Source: CAD feature listing. Evaluate the final solid. Frame: model axes, mm. Face numbers are marked on the shaded views. Coordinates: 2 decimals unless noted, no trailing zeros. Loops run counter-clockwise (first coordinate to the right, second up) from the corner with the lowest first, then second, coordinate; pieces in that order, holes last. Notation, with made-up numbers: M 41.25,74.5 L 60.25,74.5 A18 cw 60.25,81.5 Z; hole C 42.5,-36.5 d3. An arc over 180 degrees is marked long. One line per question, with ' | ' between items. Start each with the question number.
1. Mould query, pull axis Y, two halves, no side actions, for the marked faces 1, 2 and 3. Classes: pulls with the +Y half, pulls with the -Y half, needs draft (parallel to the pull), parting line crosses it, or undercut.
2. Section query B-B, the plane y = 136. Output: boundary loops of the cut face in (x, z).
3. Ray query, probe 1 along Z at (x, y) = (2, 156); probe 2 along X at (y, z) = (58.5, 8.5); probe 3 along Z at (x, y) = (-29.5, 100). Return the intervals inside material, ascending.
4. Pin query (flat end, axial travel): P1, Ø1.5, axis at x = 0.5, z = -1, coming from the -Y side; P2, Ø15, axis at x = 5.5, z = -7.5, coming from the -Y side; P3, Ø4, axis at x = 4.5, y = 189, coming from the +Z side. Return the tip coordinate at first contact, or that it passes through.
5. Section query A-A, the plane y = 266. Output: boundary loops of the cut face in (x, z), and give its area (3 significant figures).
Autodesk Inventor part; units mm, degrees
ref_plane "YZ Plane" through (0, 0, 0) normal (1, 0, 0) x (0, 1, 0)
ref_plane "XZ Plane" through (0, 0, 0) normal (0, 1, 0) x (-1, 0, 0)
ref_plane "XY Plane" through (0, 0, 0) normal (0, 0, 1) x (1, 0, 0)
sketch "Boceto1" plane through (0, 0, 0) normal (0, 0, 1) x (1, 0, 0)
  point P0 (0, 0)
sketch "Boceto2" plane through (0, 0, 0) normal (0, 1, 0) x (-1, 0, 0)
  point P0 (0, 0)
sketch "Boceto3" plane through (0, 0, 0) normal (0, 1, 0) x (-1, 0, 0)
  circle A0 centre (0, 0) radius 37.5
  dimension "d0" = 75
extrude "Extrusión1" add sketch "Boceto3" along normal blind 190
sketch "Boceto4" plane through (0, 190, 0) normal (0, 1, 0) x (1, 0, 0)
  circle A0 centre (0, 0) radius 14
  dimension "d3" = 28
extrude "Extrusión2" add sketch "Boceto4" along normal blind 95
fillet "Empalme1" radius 30 1 edges at (-14, 190, 0)
fillet "Empalme2" radius 30 2 edges at (0, 190, -37.5) (0, 190, 37.5)
sketch "Boceto5" plane through (0, 285, 0) normal (0, 1, 0) x (1, 0, 0)
  circle A0 centre (0, 0) radius 15
  dimension "d8" = 30
extrude "Extrusión3" add sketch "Boceto5" along normal blind 8
sketch "Boceto6" plane through (0, 293, 0) normal (0, 1, 0) x (1, 0, 0)
  circle A0 centre (0, 0) radius 14
extrude "Extrusión4" add sketch "Boceto6" along normal blind 4
sketch "Boceto7" plane through (0, 0, 0) normal (0, -1, 0) x (1, 0, 0)
  circle A0 centre (0, 0) radius 2.5
  dimension "d13" = 5
extrude "Extrusión5" cut sketch "Boceto7" against normal blind 18
fillet "Empalme3" radius 30 1 edges at (-2.5, 0, 0)
properties part number "Botella_Vino"
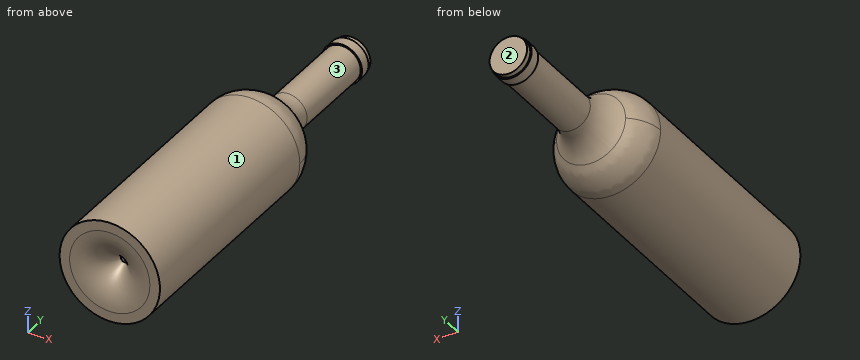
Taken from the geometry:
1) face 1: needs draft | face 2: pulls with the +Y half | face 3: undercut
2) outline: C 0,0 d75
3) probe 1: -37.45 to 37.45 | probe 2: -36.52 to 36.52 | probe 3: -23.15 to 23.15
4) P1: y = 18 | P2: y = 3.06 | P3: z = 33.01
5) outline: C 0,0 d28 | area: 616 mm^2
